Input: part model. Units: mm. Frame: model coordinates. A direction names the side the tool comes from. Give positions to 0.01 mm unless a question says otherwise; leave off trailing zeros. Write each loop counter-clockwise with the first axis right and the second up, starting at its lowest first coordinate (ties: lowest second). Pieces come first, ordered by that corner, then holes. Notation, with made-up numbers: (56.5, -9) -> (104.5, -9) arc R15 ccw to (104.5, -4) -> close; hole circle Ø7 at (42.5, 48.5). An arc over 180 degrees is marked (long way). Return JSON: item names as keys, results as strings. Group by question number.
Item 1: Section A-A, the plane x = 120. Return loops of the section in (y, z) (3 decimals), then the cut area to 3 significant figures.
Item 2: Set-up query: faces 1 (the face through (-108, -48.675, -1)), 2 (the face through (21, -52, -3.2)). Return all of +Z, -Z, +X, -X, +Y, -Y with unobstructed straight access to the full face (end or side cutting, diameter ignored); none if empty.
Item 3: Section B-B, the plane y = 9. Return loops of the section in (x, z) (3 decimals), then the cut area to 4 significant figures.
Item 4: Pin query (flat end, axial travel): P1, Ø3, axis at x = -145.925, y = -50.675, coming from the -Z side. Return the tip coordinate at first contact, or that it passes through.
Item 5: Mould query, pull axis Y, two halves, no side actions, for faces 3 (the face through (-124, 48.675, -1)), 4 (the face through (-1, -52, 6.8)). Classes: released by +Y, released by -Y, zero draft, split by the parting line, or undercut.
Item 6: Line query: line 1 (X direction, y = -22, z = -1.5) (3 decimals); line 2 (Y direction, x = 89.5, z = 1) (3 decimals); line 3 (X direction, y = 23.5, z = 3) (3 decimals). Output: solid intervals per line, ascending. Write a range as [from, to].
from build123d import *

# Parameters (mm, degrees)
SKETCH004_W       = 298.85
SKETCH004_H       = 108.35
PAD002_DEPTH      = 6.8
PAD002_DEPTH_BACK = 3.2
SKETCH010_R       = 1.1
HOLE001_DEPTH     = 4.2
HOLE001_TIPS_R    = 1.1
FILLET003_R       = 3
POCKET004_DEPTH   = 5.2
FILLET005_R       = 1
CHAMFER003_SIZE   = 0.1


with BuildPart() as part:
    # Sketch004 → Pad002 (new body, two sides)
    with BuildSketch(Plane.XY) as pad002_sk:
        Rectangle(SKETCH004_W, SKETCH004_H)
        Polygon((-143.425, 48.175), (-143.425, -48.175), (86.275, -48.175), (86.275, -29.125), (143.425, -29.125), (143.425, 48.175), align=None, mode=Mode.SUBTRACT)
    extrude(amount=PAD002_DEPTH)
    extrude(pad002_sk.sketch, amount=-PAD002_DEPTH_BACK)

    # Sketch010 (on Face11 of Pad002) → Hole001 (cut)
    with BuildSketch(Plane(origin=(0, 0, -3.2), x_dir=(1, 0, 0), z_dir=(0, 0, -1))):
        with Locations((-145.925, 50.675)):
            Circle(SKETCH010_R)
        with Locations((-145.925, -50.675)):
            Circle(SKETCH010_R)
        with Locations((145.925, 50.675)):
            Circle(SKETCH010_R)
        with Locations((145.925, -50.675)):
            Circle(SKETCH010_R)
    extrude(amount=-HOLE001_DEPTH, mode=Mode.SUBTRACT)

    # Hole001 tips → Hole001 tip 1 section 0
    with BuildSketch(Plane(origin=(0, 0, 1), x_dir=(1, 0, 0), z_dir=(0, 0, -1)), mode=Mode.PRIVATE) as hole001_tip_1_s0:
        with Locations((-145.925, 50.675)):
            Circle(HOLE001_TIPS_R)
    loft([hole001_tip_1_s0.sketch, Vertex(-145.925, -50.675, 1.660947)], mode=Mode.SUBTRACT)

    # Hole001 tips → Hole001 tip 2 section 0
    with BuildSketch(Plane(origin=(0, 0, 1), x_dir=(1, 0, 0), z_dir=(0, 0, -1)), mode=Mode.PRIVATE) as hole001_tip_2_s0:
        with Locations((-145.925, -50.675)):
            Circle(HOLE001_TIPS_R)
    loft([hole001_tip_2_s0.sketch, Vertex(-145.925, 50.675, 1.660947)], mode=Mode.SUBTRACT)

    # Hole001 tips → Hole001 tip 3 section 0
    with BuildSketch(Plane(origin=(0, 0, 1), x_dir=(1, 0, 0), z_dir=(0, 0, -1)), mode=Mode.PRIVATE) as hole001_tip_3_s0:
        with Locations((145.925, 50.675)):
            Circle(HOLE001_TIPS_R)
    loft([hole001_tip_3_s0.sketch, Vertex(145.925, -50.675, 1.660947)], mode=Mode.SUBTRACT)

    # Hole001 tips → Hole001 tip 4 section 0
    with BuildSketch(Plane(origin=(0, 0, 1), x_dir=(1, 0, 0), z_dir=(0, 0, -1)), mode=Mode.PRIVATE) as hole001_tip_4_s0:
        with Locations((145.925, -50.675)):
            Circle(HOLE001_TIPS_R)
    loft([hole001_tip_4_s0.sketch, Vertex(145.925, 50.675, 1.660947)], mode=Mode.SUBTRACT)

    # Fillet003
    fillet003_edges = [part.edges().sort_by_distance(p)[0] for p in [
        (149.425, 54.175, 1.8),
        (149.425, -54.175, 1.8),
        (-149.425, 54.175, 1.8),
        (-149.425, -54.175, 1.8),
    ]]
    fillet(fillet003_edges, radius=FILLET003_R)

    # Sketch011 (on Face2 of Fillet003) → Pocket004 (cut)
    with BuildSketch(Plane(origin=(0, 0, -3.2), x_dir=(1, 0, 0), z_dir=(0, 0, -1))):
        Polygon((-143.925, 48.675), (-72.4875, 48.675), (-72.4875, 51.175), (48.675, 51.175), (48.675, 48.675), (86.775, 48.675), (86.775, 29.625), (143.925, 29.625), (143.925, 10.575), (146.425, 10.575), (146.425, -29.625), (143.925, -29.625), (143.925, -48.675), (105.825, -48.675), (105.825, -51.175), (46.575, -51.175), (46.575, -48.675), (-46.575, -48.675), (-46.575, -51.175), (-105.825, -51.175), (-105.825, -48.675), (-143.925, -48.675), (-143.925, -29.625), (-146.425, -29.625), (-146.425, 29.625), (-143.925, 29.625), align=None)
    extrude(amount=-POCKET004_DEPTH, mode=Mode.SUBTRACT)

    # Fillet005
    fillet005_edges = [part.edges().sort_by_distance(p)[0] for p in [
        (146.425, -10.575, -0.6),
        (143.925, -29.625, -0.6),
        (146.425, 29.625, -0.6),
        (143.925, 48.675, -0.6),
        (105.825, 51.175, -0.6),
        (46.575, 51.175, -0.6),
        (-46.575, 51.175, -0.6),
        (-105.825, 51.175, -0.6),
        (-143.925, 48.675, -0.6),
        (-146.425, 29.625, -0.6),
        (-146.425, -29.625, -0.6),
        (-143.925, -48.675, -0.6),
        (48.675, -51.175, -0.6),
        (-72.4875, -51.175, -0.6),
        (86.775, -48.675, -0.6),
    ]]
    fillet(fillet005_edges, radius=FILLET005_R)

    # Chamfer003
    chamfer003_edges = [part.edges().sort_by_distance(p)[0] for p in [
        (0, 48.675, -3.2),
        (76.2, 51.175, -3.2),
        (143.925, 38.65, -3.2),
        (146.425, 9.525, -3.2),
        (114.85, -29.625, -3.2),
        (86.775, -38.65, -3.2),
        (-146.425, 0, -3.2),
        (-143.925, 38.65, -3.2),
        (-143.925, 29.625, -0.6),
        (-46.575, 48.675, -0.6),
        (86.775, -29.625, -0.6),
        (-72.4875, -48.675, -0.6),
        (-11.90625, -51.175, -3.2),
        (-107.70625, -48.675, -3.2),
        (48.675, -48.675, -0.6),
        (-143.925, -29.625, -0.6),
        (-105.825, 48.675, -0.6),
        (143.925, 29.625, -0.6),
        (143.925, -10.575, -0.6),
        (105.825, 48.675, -0.6),
        (46.575, 48.675, -0.6),
        (-46.575, 49.425, -3.2),
        (114.85, -29.125, 2),
        (86.275, -38.65, 2),
        (86.275, -29.125, 4.4),
        (-28.575, -48.175, 2),
        (143.425, 9.525, 2),
        (0, 48.175, 2),
        (-143.425, 0, 2),
        (-148.54632, -53.29632, -3.2),
        (148.54632, -53.29632, 6.8),
        (143.425, 9.525, 6.8),
        (114.85, -29.125, 6.8),
        (86.275, -38.65, 6.8),
        (-28.575, -48.175, 6.8),
        (0, 48.175, 6.8),
        (-143.425, 0, 6.8),
    ]]
    chamfer(chamfer003_edges, length=CHAMFER003_SIZE)


solid = part.part
Answer below:
{
 "1": {"outline": "(-54.175, -3.1) -> (-54.075, -3.2) -> (-29.725, -3.2) -> (-29.625, -3.1) -> (-29.625, 2) -> (-29.225, 2) -> (-29.125, 2.1) -> (-29.125, 6.7) -> (-29.225, 6.8) -> (-54.075, 6.8) -> (-54.175, 6.7) -> close; (48.175, 2.1) -> (48.275, 2) -> (48.675, 2) -> (48.675, -3.1) -> (48.775, -3.2) -> (54.075, -3.2) -> (54.175, -3.1) -> (54.175, 6.7) -> (54.075, 6.8) -> (48.275, 6.8) -> (48.175, 6.7) -> close", "area": "305 mm2"},
 "2": {"face 1": "-Z", "face 2": "-Z, +X, -X, +Y, -Y"},
 "3": {"outline": "(-149.425, -3.1) -> (-149.325, -3.2) -> (-146.525, -3.2) -> (-146.425, -3.1) -> (-146.425, 2) -> (-143.525, 2) -> (-143.425, 2.1) -> (-143.425, 6.7) -> (-143.525, 6.8) -> (-149.325, 6.8) -> (-149.425, 6.7) -> close; (143.425, 2.1) -> (143.525, 2) -> (146.425, 2) -> (146.425, -3.1) -> (146.525, -3.2) -> (149.325, -3.2) -> (149.425, -3.1) -> (149.425, 6.7) -> (149.325, 6.8) -> (143.525, 6.8) -> (143.425, 6.7) -> close", "area": "88.75 mm2"},
 "4": {"P1": "stops at z = -3.2"},
 "5": {"face 3": "undercut", "face 4": "zero draft"},
 "6": {"line 1": "x = [-149.425, -146.425], [143.925, 149.425]", "line 2": "y = [-54.175, -29.625], [51.175, 54.175]", "line 3": "x = [-149.425, -143.425], [143.425, 149.425]"}
}
